Here's how the part is built. I have some questions about the finished solid (model axes, mm). Give positions to 0.01 mm unless a question says otherwise; leave off trailing zeros. Loops run counter-clockwise (first coordinate to the right, second up) from the corner with the lowest first, then second, coordinate; pieces in that order, holes last. Notation, with made-up numbers: (86, 52.25) - (101, 52.25) arc R3 cw to (101, 56.25) - close; hole circle Ø8 at (-13, 73.5). An arc over 180 degrees is marked (long way). Use a Markdown table: item, result.
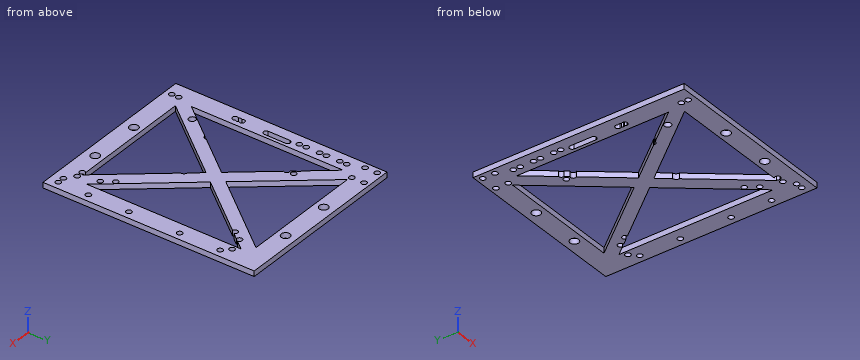
from build123d import *

# Parameters (mm, degrees)
SKETCH3_W            = 65.532
SKETCH3_H            = 78.232
SKETCH3_R            = 1
SKETCH3_R_2          = 1.25
SKETCH3_R_3          = 1.6
BOSS_EXTRUDE10_DEPTH = 2


with BuildPart() as part:
    # Sketch3 → Boss-Extrude10 (new body)
    with BuildSketch(Plane.XY):
        with Locations((-32.766, 39.116)):
            Rectangle(SKETCH3_W, SKETCH3_H)
        with Locations((-60.198, 2.535)):
            Circle(SKETCH3_R, mode=Mode.SUBTRACT)
        with Locations((-60.198, 5.075)):
            Circle(SKETCH3_R, mode=Mode.SUBTRACT)
        with Locations((-53.34, 15.24)):
            Circle(SKETCH3_R_2, mode=Mode.SUBTRACT)
        with Locations((-39.450944, 4.064)):
            Circle(SKETCH3_R_3, mode=Mode.SUBTRACT)
        with BuildLine():
            ThreePointArc((-60.547487864, 25.781), (-60.378588258, 25.483259443), (-60.32, 25.146))
            ThreePointArc((-60.32, 25.146), (-61.657259443, 24.204588258), (-62.092512136, 25.781))
            ThreePointArc((-62.092512136, 25.781), (-62.32, 26.416), (-62.092512136, 27.051))
            ThreePointArc((-62.092512136, 27.051), (-61.657259443, 28.627411742), (-60.32, 27.686))
            ThreePointArc((-60.32, 27.686), (-60.378588258, 27.348740557), (-60.547487864, 27.051))
            ThreePointArc((-60.547487864, 27.051), (-60.378588258, 26.753259443), (-60.32, 26.416))
            ThreePointArc((-60.32, 26.416), (-60.378588258, 26.078740557), (-60.547487864, 25.781))
        make_face(mode=Mode.SUBTRACT)
        with BuildLine():
            Line((-11.628420455, 7), (-56.019094707, 7))
            Line((-56.019094707, 7), (-33.112109743, 35.552384115))
            Line((-33.112109743, 35.552384115), (-29.697720228, 31.296522373))
            ThreePointArc((-29.697720228, 31.296522373), (-28.738744364, 30.752879791), (-28.359, 29.718))
            ThreePointArc((-28.359, 29.718), (-28.359594089, 29.67440261), (-28.361375915, 29.630837597))
            Line((-28.361375915, 29.630837597), (-10.205124779, 7))
            Line((-10.205124779, 7), (-10.773355545, 7))
            ThreePointArc((-10.773355545, 7), (-10.356041134, 6.631008199), (-10.200888, 6.096))
            ThreePointArc((-10.200888, 6.096), (-11.735896199, 5.251153134), (-11.628420455, 7))
        make_face(mode=Mode.SUBTRACT)
        with Locations((-20.574, 3.890944)):
            Circle(SKETCH3_R_3, mode=Mode.SUBTRACT)
        with Locations((-8.700888, 6.096)):
            Circle(SKETCH3_R, mode=Mode.SUBTRACT)
        with Locations((-5.339, 3.556)):
            Circle(SKETCH3_R, mode=Mode.SUBTRACT)
        with Locations((-2.799, 3.556)):
            Circle(SKETCH3_R, mode=Mode.SUBTRACT)
        with Locations((-10.668, 13.208)):
            Circle(SKETCH3_R, mode=Mode.SUBTRACT)
        with Locations((-13.213, 17.018)):
            Circle(SKETCH3_R, mode=Mode.SUBTRACT)
        with Locations((-2.794, 14.728)):
            Circle(SKETCH3_R, mode=Mode.SUBTRACT)
        with Locations((-2.794, 29.718)):
            Circle(SKETCH3_R, mode=Mode.SUBTRACT)
        with BuildLine():
            ThreePointArc((-61.706, 45.116), (-60.706, 46.116), (-59.706, 45.116))
            Line((-59.706, 45.116), (-59.706, 37.116))
            ThreePointArc((-59.706, 37.116), (-60.706, 36.116), (-61.706, 37.116))
            Line((-61.706, 37.116), (-61.706, 45.116))
        make_face(mode=Mode.SUBTRACT)
        with Locations((-61.722, 48.629)):
            Circle(SKETCH3_R, mode=Mode.SUBTRACT)
        with Locations((-61.722, 51.169)):
            Circle(SKETCH3_R, mode=Mode.SUBTRACT)
        with Locations((-61.722, 56.129)):
            Circle(SKETCH3_R, mode=Mode.SUBTRACT)
        with Locations((-61.722, 58.669)):
            Circle(SKETCH3_R, mode=Mode.SUBTRACT)
        with BuildLine():
            Line((-58.532, 10.995023961), (-58.532, 67.236976039))
            Line((-58.532, 67.236976039), (-50.821827001, 57.626640091))
            ThreePointArc((-50.821827001, 57.626640091), (-50.014999166, 57.252778474), (-49.824952048, 56.384086494))
            Line((-49.824952048, 56.384086494), (-48.700366603, 54.982348306))
            ThreePointArc((-48.700366603, 54.982348306), (-47.474999166, 54.712778474), (-47.477503777, 53.458112393))
            Line((-47.477503777, 53.458112393), (-35.971124779, 39.116))
            Line((-35.971124779, 39.116), (-47.320258494, 24.969885803))
            ThreePointArc((-47.320258494, 24.969885803), (-47.275179837, 24.801577784), (-47.26, 24.628))
            ThreePointArc((-47.26, 24.628), (-47.600460693, 23.876329925), (-48.390015804, 23.636488078))
            Line((-48.390015804, 23.636488078), (-58.532, 10.995023961))
        make_face(mode=Mode.SUBTRACT)
        with Locations((-48.255, 56.627)):
            Circle(SKETCH3_R, mode=Mode.SUBTRACT)
        Polygon((-32.766, 43.111023961), (-55.326875221, 71.232), (-10.205124779, 71.232), align=None, mode=Mode.SUBTRACT)
        with Locations((-61.722, 63.629)):
            Circle(SKETCH3_R, mode=Mode.SUBTRACT)
        with Locations((-61.722, 66.169)):
            Circle(SKETCH3_R, mode=Mode.SUBTRACT)
        with Locations((-63.448, 71.664)):
            Circle(SKETCH3_R, mode=Mode.SUBTRACT)
        with Locations((-63.448, 76.164)):
            Circle(SKETCH3_R, mode=Mode.SUBTRACT)
        with Locations((-56.948, 71.664)):
            Circle(SKETCH3_R, mode=Mode.SUBTRACT)
        with Locations((-56.948, 76.164)):
            Circle(SKETCH3_R, mode=Mode.SUBTRACT)
        with Locations((-39.37, 74.422)):
            Circle(SKETCH3_R_3, mode=Mode.SUBTRACT)
        with BuildLine():
            Line((-9.668009055, 64.774255485), (-7, 68.099792192))
            Line((-7, 68.099792192), (-7, 10.995023961))
            Line((-7, 10.995023961), (-29.906984964, 39.547408077))
            Line((-29.906984964, 39.547408077), (-13.321002101, 60.220986655))
            ThreePointArc((-13.321002101, 60.220986655), (-13.983000834, 61.839778474), (-12.259188179, 61.544483353))
            Line((-12.259188179, 61.544483353), (-10.455353631, 63.792870775))
            ThreePointArc((-10.455353631, 63.792870775), (-11.448000834, 65.395778474), (-9.668009055, 64.774255485))
        make_face(mode=Mode.SUBTRACT)
        with Locations((-2.794, 48.514)):
            Circle(SKETCH3_R, mode=Mode.SUBTRACT)
        with Locations((-20.574, 74.422)):
            Circle(SKETCH3_R_3, mode=Mode.SUBTRACT)
        with Locations((-2.794, 63.504)):
            Circle(SKETCH3_R, mode=Mode.SUBTRACT)
        with Locations((-5.309112, 66.04)):
            Circle(SKETCH3_R, mode=Mode.SUBTRACT)
    extrude(amount=BOSS_EXTRUDE10_DEPTH)


solid = part.part
(1) Suppose I cut it at C-C on x = -53.34. Write out the boundary of the cut face in (y, z).
A:
| item | result |
|---|---|
| outline | (0, 0) - (7, 0) - (7, 2) - (0, 2) - close; (10.34, 0) - (13.99, 0) - (13.99, 2) - (10.34, 2) - close; (16.49, 0) - (17.47, 0) - (17.47, 2) - (16.49, 2) - close; (60.77, 0) - (68.76, 0) - (68.76, 2) - (60.77, 2) - close; (71.23, 0) - (78.23, 0) - (78.23, 2) - (71.23, 2) - close |
(2) Suppose I cut it at B-B on y = 33.5. Write out the boundary of the cut face in (x, z).
A:
| item | result |
|---|---|
| outline | (-65.53, 0) - (-58.53, 0) - (-58.53, 2) - (-65.53, 2) - close; (-40.48, 0) - (-34.76, 0) - (-34.76, 2) - (-40.48, 2) - close; (-31.47, 0) - (-25.06, 0) - (-25.06, 2) - (-31.47, 2) - close; (-7, 0) - (0, 0) - (0, 2) - (-7, 2) - close |
(3) If I drill on line 1 (X direction, y = 61.5, z = 0.4); line 2 (Y direction, x = -39.37, z = 1.45); line 3 (Y direction, x = -38.5, z = 1.8), over which ranges is the centre line in solid material (lowest first)?
A:
| item | result |
|---|---|
| line 1 | -65.53 to -58.53, -53.93 to -47.52, -18.01 to -14.16, -7 to 0 |
| line 2 | 0 to 2.47, 5.66 to 7, 27.75 to 34.88, 43.35 to 51.34, 71.23 to 72.82, 76.02 to 78.23 |
| line 3 | 0 to 2.78, 5.35 to 7, 28.84 to 35.96, 42.27 to 50.26, 71.23 to 73.08, 75.76 to 78.23 |
(4) Will this pin go through, and if not, where does the flat tip stop? pin 1 (1.2 mm diameter, centred on x = -2.794, y = 48.514, fed in from +Z).
A:
| item | result |
|---|---|
| pin 1 | through |
(5) Suppose I cut it at D-D on x = -27. Write out the boundary of the cut face in (y, z), plus the area to 3 significant figures.
A:
| item | result |
|---|---|
| outline | (0, 0) - (7, 0) - (7, 2) - (0, 2) - close; (27.93, 0) - (35.92, 0) - (35.92, 2) - (27.93, 2) - close; (43.17, 0) - (50.3, 0) - (50.3, 2) - (43.17, 2) - close; (71.23, 0) - (78.23, 0) - (78.23, 2) - (71.23, 2) - close |
| area | 58.2 mm2 |
(6) Suppose I cut it at A-A on x = -39.37. Write out the boundary of the cut face in (y, z), plus the area to 3 significant figures.
A:
| item | result |
|---|---|
| outline | (0, 0) - (2.47, 0) - (2.47, 2) - (0, 2) - close; (5.66, 0) - (7, 0) - (7, 2) - (5.66, 2) - close; (27.75, 0) - (34.88, 0) - (34.88, 2) - (27.75, 2) - close; (43.35, 0) - (51.34, 0) - (51.34, 2) - (43.35, 2) - close; (71.23, 0) - (72.82, 0) - (72.82, 2) - (71.23, 2) - close; (76.02, 0) - (78.23, 0) - (78.23, 2) - (76.02, 2) - close |
| area | 45.4 mm2 |
